The model under review builds one solid part; all positions refer to its coordinate system, in mm. Face numbers are marked on the shaded views. A direction names the side the tool comes from. Give positions to 0.01 mm unless a question says otherwise; leave off trailing zeros. Order: outer loops, then holes, each group sorted by start corner. A loop starts at its lowest first (then second) coordinate and runs counter-clockwise, first axis right, second up. Notation, with made-up numbers: (10.5, 70) - (28.5, 70) arc R10 cw to (28.5, 87) - close; hole circle Ø10 at (60.5, -31). An arc over 180 degrees is marked (long way). Write item = value, one per line. Start each with the question number.
1. For P1, Ø5, axis at y = 14.5, z = 21, coming from the -X side (3 decimals); P2, Ø4, axis at y = 16.5, z = 2, coming from the +X side (3 decimals); P3, Ø3, axis at x = -11, y = -3.5, coming from the +Z side, all flat-tipped, find the tip position at first contact; note any pin that passes through.
2. Mouldability with a two-part tool opening along X and no side actions: class the marked faces 5, 6, 7 and 8 as pulls with the +X half, pulls with the -X half, needs draft (parallel to the pull), parting line crosses it, or undercut.
3. We need section A-A, the plane y = 15. Give the boundary of the cut face in (x, z) (3 decimals).
4. Wall thickness on probe 1 along Y at (x, z) = (-14.5, 12.5); probe 2 along Z at (x, y) = (34, -28) (3 decimals); probe 3 along Z at (x, y) = (93, -1) (3 decimals): over which ranges is each line inside the solid? List them lowest first.
5. Machinability: for the marked faces 1, 2, 3 and 4, which of the approach directions +Z, -Z, +X, -X, +Y, -Y give a long, thin tool a straight path to every point of the face, cutting with its end or side? Answer none if there is none.
6. We need section B-B, the plane y = 38. Give the boundary of the cut face in (x, z) (3 decimals), and give its area (3 significant figures).
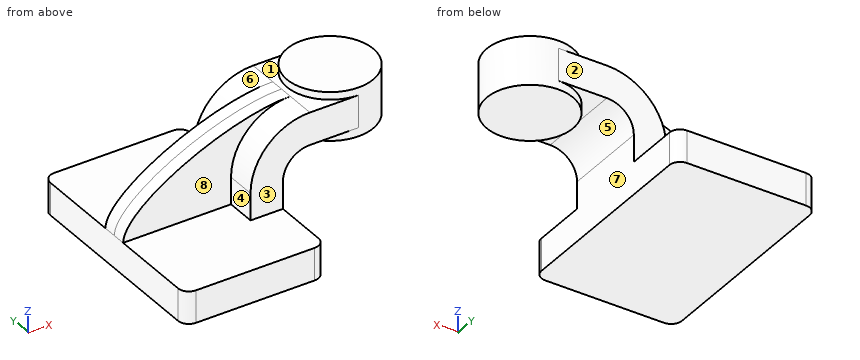
from build123d import *

# Parameters (mm, degrees)
F1_DEPTH = 63.5
F2_DEPTH = 25.4
F3_DEPTH = 7.9375
F0_W     = 25.4
F0_H     = 19.05
F4_DEPTH = 25.4
F6_R     = 6.35


with BuildPart() as f1:
    # F0 (on Front) → F1 (new body, symmetric)
    with BuildSketch(Plane.XZ):
        Polygon((-41.275, 9.525), (-41.275, -9.525), (41.275, -9.525), (41.275, 9.525), (22.225, 9.525), align=None)
    extrude(amount=F1_DEPTH, both=True)

    # F0 (on Front) → F2 (join, symmetric)
    with BuildSketch(Plane.XZ):
        with BuildLine():
            Line((22.225, 9.525), (41.275, 9.525))
            Line((41.275, 9.525), (41.275, 25.4))
            ThreePointArc((41.275, 25.4), (45.9246798487, 36.6253201513), (57.15, 41.275))
            Line((57.15, 41.275), (60.325, 41.275))
            Line((60.325, 41.275), (60.325, 60.325))
            Line((60.325, 60.325), (57.15, 60.325))
            ThreePointArc((57.15, 60.325), (32.4542956671, 50.0957043329), (22.225, 25.4))
            Line((22.225, 25.4), (22.225, 9.525))
        make_face()
    extrude(amount=F2_DEPTH, both=True)

    # F0 (on Front) → F3 (join, symmetric)
    with BuildSketch(Plane.XZ):
        with BuildLine():
            add(Edge.make_bspline(
                [(-41.275, 9.525), (-40.2447469532, 30.1753021777), (21.1324393749, 60.5111531913), (57.15, 60.325)],
                knots=[0, 0, 0, 0, 110.761548495, 110.761548495, 110.761548495, 110.761548495], degree=3))
            Line((-41.275, 9.525), (22.225, 9.525))
            Line((22.225, 9.525), (22.225, 25.4))
            ThreePointArc((22.225, 25.4), (32.4542956671, 50.0957043329), (57.15, 60.325))
        make_face()
    extrude(amount=F3_DEPTH, both=True)

    # F0 (on Front) → F4 (join, symmetric)
    with BuildSketch(Plane.XZ):
        with Locations((73.025, 50.8)):
            Rectangle(F0_W, F0_H)
    extrude(amount=F4_DEPTH, both=True)

    # F0 (on Front) → F5 (revolve)
    with BuildSketch(Plane.XZ):
        Polygon((85.725, 64.77), (85.725, 60.325), (85.725, 41.275), (85.725, 36.195), (111.125, 36.195), (111.125, 64.77), align=None)
    revolve(axis=Axis((85.725, 0, 50.8), (0, 0, -1)))

    # F6
    f6_edges = [f1.edges().sort_by_distance(p)[0] for p in [
        (41.275, -63.5, 0),
        (-41.275, -63.5, 0),
        (41.275, 63.5, 0),
        (-41.275, 63.5, 0),
    ]]
    fillet(f6_edges, radius=F6_R)


solid = f1.part
Model answer:
q1.P1 = 22.225
q1.P2 = 41.275
q1.P3 = 40.47
q2.face_5 = undercut
q2.face_6 = pulls with the -X half
q2.face_7 = pulls with the +X half
q2.face_8 = needs draft
q3.outline = (-41.275, -9.525) - (41.275, -9.525) - (41.275, 25.4) arc R15.875 cw to (57.15, 41.275) - (65.227, 41.275) - (65.227, 36.195) - (106.223, 36.195) - (106.223, 64.77) - (65.227, 64.77) - (65.227, 60.325) - (57.15, 60.325) arc R34.925 ccw to (22.225, 25.4) - (22.225, 9.525) - (-41.275, 9.525) - close
q4.probe_1 = -7.94 to 7.94
q4.probe_2 = -9.525 to 9.525
q4.probe_3 = 36.195 to 64.77
q5.face_1 = +Z, -X
q5.face_2 = +Z, +X, -X, +Y
q5.face_3 = +Z, +X, -X, -Y
q5.face_4 = +Z, -X, -Y
q6.outline = (-41.275, -9.525) - (41.275, -9.525) - (41.275, 9.525) - (-41.275, 9.525) - close
q6.area = 1,570 mm2
